The listing builds one solid part. Answer for the finished solid, in the listing's coordinates (mm). Face numbers are marked on the shaded views. A direction names the side the tool comes from. Coordinates: 2 decimals unless noted, no trailing zeros. Loops run counter-clockwise (first coordinate to the right, second up) from the corner with the lowest first, then second, coordinate; pieces in that order, holes last. Notation, with made-up numbers: (-13.75, -18) - (-1.75, -18) arc R31 ccw to (-1.75, 17) - close; hole circle Ø7 at (30, 36). An arc over 180 degrees is marked (long way). One line per question, with ' | ' between items.
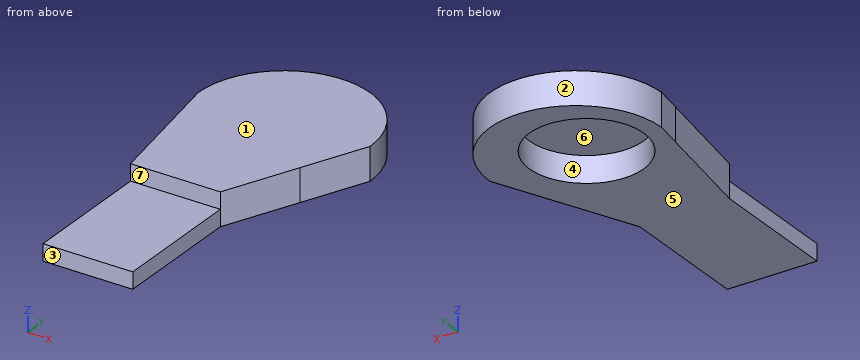
from build123d import *

# Parameters (mm, degrees)
F1_DEPTH = 25
F2_R     = 43.2644605555
F3_DEPTH = 20
F4_W     = 100
F4_H     = 12.5
F5_DEPTH = 113.2522414455


with BuildPart() as f1:
    # F0 (on Top) → F1 (new body)
    with BuildSketch(Plane.XY):
        with BuildLine():
            Line((43.8576357287, -47.9740324372), (65, 0))
            ThreePointArc((65, 0), (0, 65), (-65, 0))
            Line((-65, 0), (-61.6307134035, -20.655632776))
            ThreePointArc((-61.6307134035, -20.655632776), (-16.2955304461, -62.9242058947), (43.8576357287, -47.9740324372))
        make_face()
        with BuildLine():
            Line((19.7487585545, -102.6793643832), (43.8576357287, -47.9740324372))
            ThreePointArc((43.8576357287, -47.9740324372), (-16.2955304461, -62.9242058947), (-61.6307134035, -20.655632776))
            Line((-61.6307134035, -20.655632776), (-48.2512414455, -102.6793643832))
            Line((-48.2512414455, -102.6793643832), (-48.2512414455, -202.6793643832))
            Line((-48.2512414455, -202.6793643832), (19.7487585545, -202.6793643832))
            Line((19.7487585545, -202.6793643832), (19.7487585545, -102.6793643832))
        make_face()
    extrude(amount=F1_DEPTH)

    # F2 (on face) → F3 (cut)
    with BuildSketch(Plane(origin=(0, 0, 0), x_dir=(1, 0, 0), z_dir=(0, 0, -1))):
        with Locations((-8.1178825349, 0)):
            Circle(F2_R)
    extrude(amount=-F3_DEPTH, mode=Mode.SUBTRACT)

    # F4 (on face) → F5 (cut, through all)
    with BuildSketch(Plane(origin=(-48.2512414455, 0, 0), x_dir=(0, -1, 0), z_dir=(-1, 0, 0))):
        with Locations((152.6793643832, 18.75)):
            Rectangle(F4_W, F4_H)
    extrude(amount=-F5_DEPTH, mode=Mode.SUBTRACT)


solid = f1.part
Item 1: Which of the six approach directions +Z, -Z, +X, -X, +Y, -Y give full straight-line access (tool end or side, diameter ignored) to the marked faces 5, 6 and 7?
Taken from the geometry:
face 5: -Z, +X, -X, +Y, -Y | face 6: -Z | face 7: +Z, +X, -X, -Y
Item 2: The mould has two halves that part along Y. Classify the marked faces 1, 2, 3 and 4: pulls with the +Y half, pulls with the -Y half, needs draft (parallel to the pull), parting line crosses it, or undercut.
Taken from the geometry:
face 1: needs draft | face 2: pulls with the +Y half | face 3: pulls with the -Y half | face 4: undercut
Item 3: Find section A-A, the plane z = 15.5. Write down the section's boundary in (x, y), plus the area to 3 significant figures.
Taken from the geometry:
outline: (-65, 0) - (-48.25, -102.68) - (19.75, -102.68) - (65, 0) arc R65 ccw to start; hole circle Ø86.53 at (-8.12, 0) | area: 10,900 mm2
Item 4: Find section B-B, the plane x = 14.5. Write down the section's boundary in (y, z).
Taken from the geometry:
outline: (-202.68, 0) - (-36.88, 0) - (-36.88, 20) - (36.88, 20) - (36.88, 0) - (63.36, 0) - (63.36, 25) - (-102.68, 25) - (-102.68, 12.5) - (-202.68, 12.5) - close
Item 5: Each of these flat-tipped pins is pushed along its axis until it touches: pin 1 Ø4 at (x, y) = (-43, -159) entering from -Z; pin 2 Ø4 at (x, z) = (23.5, 11.5) entering from -Y; pin 3 Ø5 at (x, z) = (44, 6.5) entering from -Y; pin 4 Ø14 at (y, z) = (-150, 3) entering from +X. Where does it stop, or does it pass through?
Taken from the geometry:
pin 1: stops at z = 0 | pin 2: stops at y = -98.71 | pin 3: stops at y = -53.32 | pin 4: stops at x = 19.75
Item 6: Find section C-C, the plane y = -115. Write down the section's boundary in (x, z).
Taken from the geometry:
outline: (-48.25, 0) - (19.75, 0) - (19.75, 12.5) - (-48.25, 12.5) - close
Item 7: Find section D-D, the plane x = 0. Write down the section's boundary in (y, z), plus the area to 3 significant figures.
Taken from the geometry:
outline: (-202.68, 0) - (-42.5, 0) - (-42.5, 20) - (42.5, 20) - (42.5, 0) - (65, 0) - (65, 25) - (-102.68, 25) - (-102.68, 12.5) - (-202.68, 12.5) - close | area: 3,740 mm2
Item 8: Find the intervals of material crossed by line 1 (Z direction, x = -46, y = -147.5); line 2 (Y direction, x = -35, z = 14); line 3 (X direction, y = -151, z = 5.75), in increasing order. Write a range as [from, to].
Taken from the geometry:
line 1: z = [0, 12.5] | line 2: y = [-102.68, -33.9], [33.9, 54.77] | line 3: x = [-48.25, 19.75]
